from build123d import *

# Parameters (mm, degrees)
F1_DEPTH = 76.2
F2_W     = 37.0748843998
F2_H     = 14.9495508522
F3_DEPTH = 25.4
F4_SIZE  = 5.08
F5_R     = 5.08


with BuildPart() as f1:
    # F0 (on Front) → F1 (new body)
    with BuildSketch(Plane.XZ):
        with BuildLine():
            ThreePointArc((0, 0), (-86.7210244843, 35.9210244843), (-50.8, -50.8))
            Line((-50.8, -50.8), (50.8, -50.8))
            ThreePointArc((50.8, -50.8), (86.7210244843, 35.9210244843), (0, 0))
        make_face()
    extrude(amount=F1_DEPTH)

    # F2 (on face) → F3 (join)
    with BuildSketch(Plane.XZ.offset(76.2)):
        with Locations((-47.2405822948, 7.4747754261)):
            Rectangle(F2_W, F2_H)
    extrude(amount=F3_DEPTH)

    # F4
    f4_edges = [f1.edges().sort_by_distance(p)[0] for p in [
        (-47.240582, -101.6, 14.949551),
        (-65.778024, -101.6, 7.474775),
        (-47.240582, -101.6, 0),
        (-28.70314, -101.6, 7.474775),
    ]]
    chamfer(f4_edges, length=F4_SIZE)

    # F5
    f5_edges = [f1.edges().sort_by_distance(p)[0] for p in [
        (-47.240582, -96.52, 0),
        (-65.778024, -96.52, 7.474775),
        (-47.240582, -96.52, 14.949551),
        (-28.70314, -96.52, 7.474775),
    ]]
    fillet(f5_edges, radius=F5_R)


solid = f1.part
Input: part model. Units: mm. Frame: model coordinates. A direction names the side the tool comes from. Give positions to 0.01 mm unless a question says otherwise; leave off trailing zeros. Order: outer loops, then holes, each group sorted by start corner. A loop starts at its lowest first (then second) coordinate and runs counter-clockwise, first axis right, second up. Notation, with made-up numbers: M 64.25,9.5 L 84.25,9.5 A29 ccw 84.25,34.5 Z; hole C 62.5,4 d8. An arc over 180 degrees is marked long. Answer as a JSON object with one key per item and string values.
1. Cut plane A-A, the plane z = 18. Output: boundary loops of the cut face in (x, y), and give its area (3 significant figures).
Result sheet:
{"outline": "M -98.3,-76.2 L -3.3,-76.2 L -3.3,0 L -98.3,0 Z; M 3.3,-76.2 L 98.3,-76.2 L 98.3,0 L 3.3,0 Z", "area": "14,500 mm²"}
2. First-contact query: P1, Ø16.5, axis at y = -88, z = 5, coming from the +X side; P2, Ø3, axis at y = -27.5, z = 37.5, coming from the +X side; P3, Ø4.5, axis at y = -81, z = 7, coming from the -X side. Flat tips, straight axial feed; report the tip coordinate or a pass-through.
Result sheet:
{"P1": "x = -28.7", "P2": "x = 86.64", "P3": "x = -65.78"}
3. Ray query, line 1 (Y direction, x = 86.5, z = 9); line 2 (X direction, y = -67, z = 4); line 3 (X direction, y = -36, z = 39.5). Return the intervals inside material, ascending. Write a range as [from, to].
Result sheet:
{"line 1": "[-76.2, 0]", "line 2": "[-101.44, -0.16], [0.16, 101.44]", "line 3": "[-82.74, -18.86], [18.86, 82.74]"}
4. Cut plane D-D, the plane x = -24. Output: boundary loops of the cut face in (y, z).
Result sheet:
{"outline": "M -76.2,-50.8 L 0,-50.8 L 0,43.16 L -76.2,43.16 Z"}
5. Cut plane C-C, the plane x = 78. Output: boundary loops of the cut face in (y, z), and give its area (3 significant figures).
Result sheet:
{"outline": "M -76.2,-42.9 L 0,-42.9 L 0,42.9 L -76.2,42.9 Z", "area": "6,540 mm²"}
6. Reachability of faces 5 (the flat face through (-48, -85, 0)), 6 (the flat face through (-1, 0, 1)), 7 (the flat face through (-48, -85, 14.95)) from +Z, -Z, +X, -X, +Y, -Y: full face, straight path, thin tool, end or side. Return the list, or none.
Result sheet:
{"face 5": "-Z, +X, -X, -Y", "face 6": "+Z, -Z, +X, -X, +Y", "face 7": "+Z, +X, -X, -Y"}
7. Cut plane B-B, the plane y = -35. Output: boundary loops of the cut face in (x, z).
Result sheet:
{"outline": "M -50.8,-50.8 L 50.8,-50.8 A50.8 ccw long 0,0 A50.8 ccw long Z"}
8. Pull-direction query (X, two-part tool) for faces 1 (the cylindrical face through (-85.5, -37.6, 37.1)), 2 (the flat face through (-65.778, -85, 7)), 3 (the flat face through (-1, -76.2, 1)), 4 (the flat face through (-28.703, -85, 7)); classes: +X half, -X half, draft (parallel to the pull), parting line (faces both ways), or undercut.
Result sheet:
{"face 1": "undercut", "face 2": "-X half", "face 3": "draft", "face 4": "+X half"}
